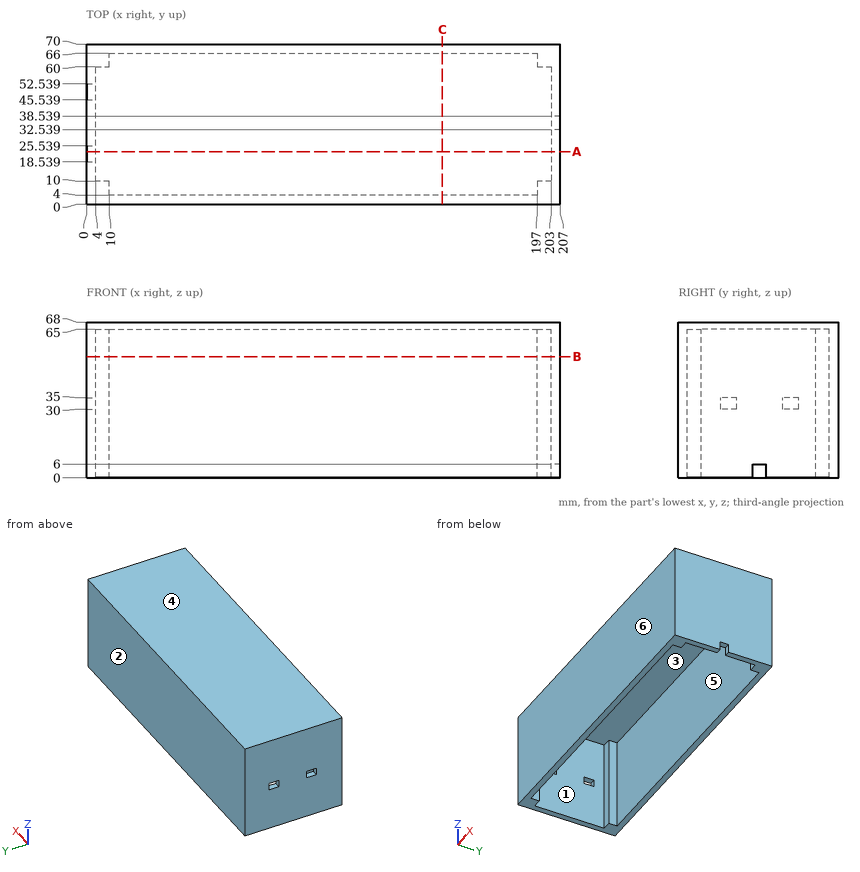
Here's the drawing with two shaded views (mm, measured from the low corner). I have some questions. A direction names the side the tool comes from. Round coordinates to 2 decimals unless told otherwise and drop trailing zeros. Write each loop counter-clockwise with the first axis right and the second up, starting at its lowest first coordinate (ties: lowest second). Pieces come first, ordered by that corner, then holes.
(1) For pin 1 (6 mm diameter, centred on x = 171, z = 38.5, fed in from -Y), with a flat end and sliding along its axis, tell me the tip position at first contact or that it passes through.
Findings below:
pin 1: stops at y = 0
(2) Which directions (+Z, -Z, +X, -X, +Y, -Y) give clear straight access to the entire face, cutting with the end or side of a thin tool? Please do the marked faces 1 and 2.
Findings below:
face 1: -Z
face 2: +Z, -Z, +X, -X, +Y
(3) Suppose I cut it at C-C on x = 155.5. Write out the boundary of the cut face in (y, z), and give its area (3 significant figures).
Findings below:
outline: (0, 0) - (4, 0) - (4, 65) - (66, 65) - (66, 0) - (70, 0) - (70, 68) - (0, 68) - close
area: 730 mm2
(4) If I drill on probe 1 along X at (y, z) = (51.5, 25); probe 2 along X at (y, z) = (7.5, 54.5); probe 3 along Y at (x, z) = (122, 27), over which ranges is the centre line in solid material (lowest first)?
Findings below:
probe 1: x = 0 to 4, 203 to 207
probe 2: x = 0 to 10, 197 to 207
probe 3: y = 0 to 4, 66 to 70
(5) Suppose I cut it at B-B on z = 53. Write out the boundary of the cut face in (x, y), and give its area (3 significant figures).
Findings below:
outline: (0, 0) - (207, 0) - (207, 70) - (0, 70) - close; hole (4, 10) - (10, 10) - (10, 4) - (197, 4) - (197, 10) - (203, 10) - (203, 60) - (197, 60) - (197, 66) - (10, 66) - (10, 60) - (4, 60) - close
area: 2,300 mm2
(6) Thinking about a two-plate mould opening in Y: for the marked faces 3, 4, 5 and 6, which applies, +Y half, -Y half, draft (parallel to the pull), parting line (faces both ways), or undercut?
Findings below:
face 3: undercut
face 4: draft
face 5: undercut
face 6: -Y half
(7) Suppose I cut it at A-A on y = 23. Write out the boundary of the cut face in (x, z).
Findings below:
outline: (0, 0) - (4, 0) - (4, 30) - (0, 30) - close; (0, 35) - (4, 35) - (4, 65) - (203, 65) - (203, 0) - (207, 0) - (207, 68) - (0, 68) - close
